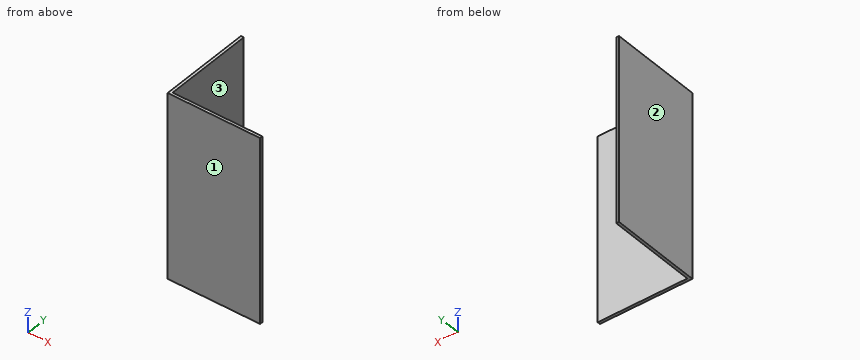
```python
from build123d import *

# Parameters (mm, degrees)
F0_W     = 600
F0_H     = 1200
F1_DEPTH = 18
F2_W     = 582
F2_H     = 1200
F3_DEPTH = 18


with BuildPart() as f1:
    # F0 (on Front) → F1 (new body)
    with BuildSketch(Plane.XZ):
        with Locations((300, 600)):
            Rectangle(F0_W, F0_H)
    extrude(amount=-F1_DEPTH)

    # F2 (on face) → F3 (join)
    with BuildSketch(Plane(origin=(0, 0, 0), x_dir=(0, -1, 0), z_dir=(-1, 0, 0))):
        with Locations((-309, 600)):
            Rectangle(F2_W, F2_H)
    extrude(amount=-F3_DEPTH)


solid = f1.part
```
Verification items for the finished model (mm, model axes). Face numbers are marked on the shaded views. Round coordinates to 2 decimals unless told otherwise and drop trailing zeros. Order: outer loops, then holes, each group sorted by start corner. A loop starts at its lowest first (then second) coordinate and runs counter-clockwise, first axis right, second up.
1) Cross-section at B-B, the plane y = 375. Record the cut outline in (x, z).
Geometry says:
outline: (0, 0) - (18, 0) - (18, 1200) - (0, 1200) - close
2) Depth check by flat-ended pin: pin 1 (1.5 mm diameter, centred on x = 227.5, z = 979, fed in from +Y); pin 2 (3 mm diameter, centred on y = 424, z = 720.5, fed in from +X). Enter the tip coordinate at first touch or a pass-through.
Geometry says:
pin 1: stops at y = 18
pin 2: stops at x = 18
3) Cross-section at A-A, the plane z = 1003. Record the cut outline in (x, y).
Geometry says:
outline: (0, 0) - (600, 0) - (600, 18) - (18, 18) - (18, 600) - (0, 600) - close
4) Material ranges on line 1 (X direction, y = 499.5, z = 397.5), recorded low to high.
Geometry says:
line 1: x = 0 to 18
5) Draft check along X on the marked faces 1, 2 and 3. Enter one of: +X half, -X half, draft (parallel to the pull), parting line (faces both ways), or undercut.
Geometry says:
face 1: draft
face 2: -X half
face 3: +X half
